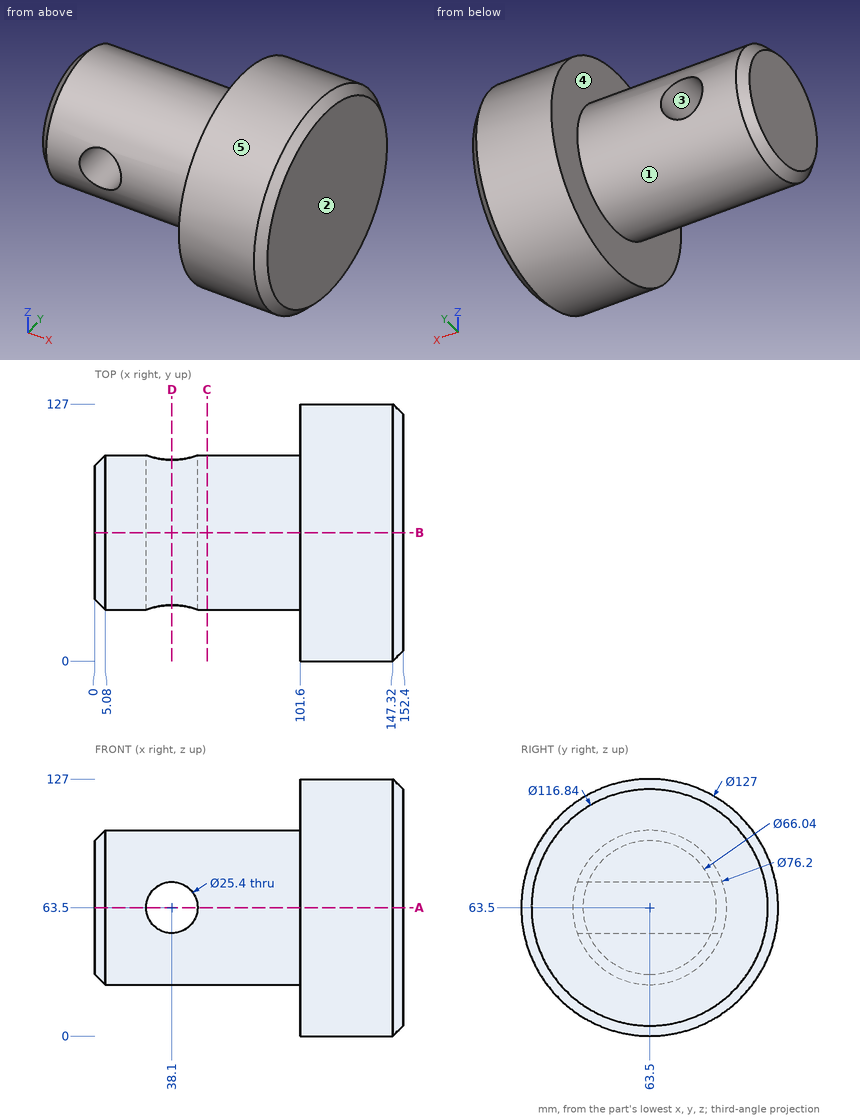
Here's the drawing with two shaded views (mm, measured from the low corner). I have some questions. A direction names the side the tool comes from. Coordinates: 2 decimals unless noted, no trailing zeros. Loops run counter-clockwise (first coordinate to the right, second up) from the corner with the lowest first, then second, coordinate; pieces in that order, holes last. Notation, with made-up numbers: M 28.5,5.25 L 87.5,5.25 A10 ccw 87.5,17.25 Z; hole C -9,85 d6. An arc over 180 degrees is marked long. Put each result on its own line as item: value. Start each with the question number.
(1) We'd pull the mould along X, two halves only. Please class the marked faces 3, 4 and 5: +X half, -X half, draft (parallel to the pull), parting line (faces both ways), or undercut.
(2) Imagine slicing it at B-B on y = 63.5. List the corners of the cut face in (x, z) for me, and give its area (3 significant figures).
(3) Imagine slicing it at A-A on z = 63.5. List the corners of the cut face in (x, y) for me, and give its area (3 significant figures).
(4) I need wall thicknesses on probe 1 along X at (y, z) = (84, 63.5); probe 2 along X at (y, z) = (111.5, 82.5); probe 3 along Y at (x, z) = (57, 62). Which ranges of each line are inside material? Lowest first, please.
(5) Imagine slicing it at C-C on x = 55.5. List the corners of the cut face in (y, z) for me, and give its area (3 significant figures).
(6) Will these pins go through, and if not, where does the flat tip stop? pin 1 Ø1 at (x, y) = (102, 71.5) entering from +Z; pin 2 Ø1 at (x, y) = (95, 35) entering from +Z; pin 3 Ø3 at (x, y) = (102, 91.5) entering from -Z; pin 4 Ø23 at (x, z) = (38.1, 63.5) entering from -Y.
(7) Which directions (+Z, -Z, +X, -X, +Y, -Y) give clear straight access to the entire face, cutting with the end or side of a thin tool? Please do the marked faces 1 and 2.
(8) Imagine slicing it at D-D on x = 38.1. List the corners of the cut face in (y, z) for me.
Worked answers:
1. face 3: undercut
1. face 4: -X half
1. face 5: draft
2. outline: M 0,30.48 L 5.08,25.4 L 101.6,25.4 L 101.6,0 L 147.32,0 L 152.4,5.08 L 152.4,121.92 L 147.32,127 L 101.6,127 L 101.6,101.6 L 5.08,101.6 L 0,96.52 Z; hole C 38.1,63.5 d25.4
2. area: 13,600 mm2
3. outline: M 0,30.48 L 5.08,25.4 L 25.4,25.4 L 25.4,101.6 L 5.08,101.6 L 0,96.52 Z; M 50.8,25.4 L 101.6,25.4 L 101.6,0 L 147.32,0 L 152.4,5.08 L 152.4,121.92 L 147.32,127 L 101.6,127 L 101.6,101.6 L 50.8,101.6 Z
3. area: 12,200 mm2
4. probe 1: x = 0 to 25.4, 50.8 to 152.4
4. probe 2: x = 101.6 to 152.4
4. probe 3: y = 25.43 to 101.57
5. outline: C 63.5,63.5 d76.2
5. area: 4,560 mm2
6. pin 1: stops at z = 126.56
6. pin 2: stops at z = 89.34
6. pin 3: stops at z = 5.79
6. pin 4: passes through
7. face 1: -X
7. face 2: +Z, -Z, +X, +Y, -Y
8. outline: M 27.58,50.8 A38.1 ccw 99.42,50.8 Z; M 27.58,76.2 L 99.42,76.2 A38.1 ccw Z
